```python
from build123d import *

# Parameters (mm, degrees)
SKETCH1_W           = 50.8
SKETCH1_H           = 50.8
BOSS_EXTRUDE1_DEPTH = 4.572
SKETCH2_R           = 8.73125
CUT_EXTRUDE7_DEPTH  = 5.572
SKETCH5_R           = 1.5875
CUT_EXTRUDE8_DEPTH  = 5.572
SKETCH7_R           = 1.5875
CUT_EXTRUDE9_DEPTH  = 5.572


with BuildPart() as part:
    # Sketch1 → Boss-Extrude1 (new body)
    with BuildSketch(Plane.XY):
        with Locations((25.4, 25.4)):
            Rectangle(SKETCH1_W, SKETCH1_H)
    extrude(amount=BOSS_EXTRUDE1_DEPTH)

    # Sketch2 → Cut-Extrude7 (cut, through all)
    with BuildSketch(Plane(origin=(0, 0, 0), x_dir=(-1, 0, 0), z_dir=(0, 0, -1))):
        with Locations((-25.4, 25.4)):
            Circle(SKETCH2_R)
    extrude(amount=-CUT_EXTRUDE7_DEPTH, mode=Mode.SUBTRACT)

    # Sketch5 → Cut-Extrude8 (cut, through all)
    with BuildSketch(Plane.XY.offset(4.572)):
        with Locations((25.4, 6.35)):
            Circle(SKETCH5_R)
        with Locations((6.35, 25.4)):
            Circle(SKETCH5_R)
        with Locations((25.4, 44.45)):
            Circle(SKETCH5_R)
        with Locations((44.45, 25.4)):
            Circle(SKETCH5_R)
    extrude(amount=-CUT_EXTRUDE8_DEPTH, mode=Mode.SUBTRACT)

    # Sketch7 → Cut-Extrude9 (cut, through all)
    with BuildSketch(Plane(origin=(0, 0, 0), x_dir=(-1, 0, 0), z_dir=(0, 0, -1))):
        with Locations((-6.35, 6.35)):
            Circle(SKETCH7_R)
        with Locations((-44.45, 6.35)):
            Circle(SKETCH7_R)
        with Locations((-44.45, 44.45)):
            Circle(SKETCH7_R)
        with Locations((-6.35, 44.45)):
            Circle(SKETCH7_R)
    extrude(amount=-CUT_EXTRUDE9_DEPTH, mode=Mode.SUBTRACT)


solid = part.part
```
Source: CAD feature listing. Evaluate the final solid. Frame: model axes, mm. Round coordinates to 2 decimals unless told otherwise and drop trailing zeros. Loops run counter-clockwise (first coordinate to the right, second up) from the corner with the lowest first, then second, coordinate; pieces in that order, holes last. Notation, with made-up numbers: M 58.5,-27 L 102.5,-27 A24 ccw 102.5,11 Z; hole C -39,27 d4. An arc over 180 degrees is marked long. Use a Markdown table: item, result. Add a question column.
1. Contact query for a flat-ended pin moving along its axis: pin 1 (1.9 mm diameter, centred on x = 6.35, y = 6.35, fed in from -Z). Output: stop coordinate, or through.
2. Pull-direction query (X, two-part tool) for faces 1 (the cylindrical face through (26.13, 43.04, 2.32)), 2 (the flat face through (0, 25, 2)), 3 (the flat face through (25, 50.8, 2)); classes: +X half, -X half, draft (parallel to the pull), parting line (faces both ways), or undercut.
3. Cut plane B-B, the plane x = 44.45. Output: boundary loops of the cut face in (y, z).
4. Cut plane D-D, the plane x = 30.5. Output: boundary loops of the cut face in (y, z).
5. Cut plane C-C, the plane y = 32.5. Output: boundary loops of the cut face in (x, z).
6. Ray query, line 1 along Y through (x, z) = (44.45, 1.5); line 2 along Y through (x, z) = (25.4, 3.2). Return the intervals inside material, ascending. Write a range as [from, to].
7. Cut plane A-A, the plane y = 25.4. Output: boundary loops of the cut face in (x, z), and give its area (3 significant figures).
Solution:
| question | item | result |
|---|---|---|
| 1 | pin 1 | passes through |
| 2 | face 1 | undercut |
| 2 | face 2 | -X half |
| 2 | face 3 | draft |
| 3 | outline | M 0,0 L 4.76,0 L 4.76,4.57 L 0,4.57 Z; M 7.94,0 L 23.81,0 L 23.81,4.57 L 7.94,4.57 Z; M 26.99,0 L 42.86,0 L 42.86,4.57 L 26.99,4.57 Z; M 46.04,0 L 50.8,0 L 50.8,4.57 L 46.04,4.57 Z |
| 4 | outline | M 0,0 L 18.31,0 L 18.31,4.57 L 0,4.57 Z; M 32.49,0 L 50.8,0 L 50.8,4.57 L 32.49,4.57 Z |
| 5 | outline | M 0,0 L 20.32,0 L 20.32,4.57 L 0,4.57 Z; M 30.48,0 L 50.8,0 L 50.8,4.57 L 30.48,4.57 Z |
| 6 | line 1 | y = [0, 4.76], [7.94, 23.81], [26.99, 42.86], [46.04, 50.8] |
| 6 | line 2 | y = [0, 4.76], [7.94, 16.67], [34.13, 42.86], [46.04, 50.8] |
| 7 | outline | M 0,0 L 4.76,0 L 4.76,4.57 L 0,4.57 Z; M 7.94,0 L 16.67,0 L 16.67,4.57 L 7.94,4.57 Z; M 34.13,0 L 42.86,0 L 42.86,4.57 L 34.13,4.57 Z; M 46.04,0 L 50.8,0 L 50.8,4.57 L 46.04,4.57 Z |
| 7 | area | 123 mm2 |
